Autodesk Inventor part; units mm, degrees
ref_plane "Arbeitsebene2" through (0, 0, 0) normal (1, 0, 0) x (0, 0, -1)
ref_plane "YZ Plane" through (0, 0, 0) normal (1, 0, 0) x (0, 1, 0)
ref_plane "XY Plane" through (0, 0, 0) normal (0, 0, 1) x (1, 0, 0)
sketch "Skizze1" plane through (0, 0, 0) normal (1, 0, 0) x (0, 1, 0)
  line L0 (-11, 0) -> (-6, 0)
  arc A0 (6, 0) -> (-6, 0) centre (0, 0) ccw
  line L1 (6, 0) -> (11, 0)
  line L2 (11, 0) -> (11, 8)
  line L3 (-11, 8) -> (-11, 0)
  line L4 (-11, 8) -> (11, 8)
  point P0 (0, 0)
  dimension "d2" = 6
  dimension "d18" = 22
  dimension "d26" = 8
extrude "Extrusion1" add sketch "Skizze1" along normal mid plane 5
ref_plane "Arbeitsebene2" through (0, 0, 0) normal (1, 0, 0) x (0, 0, -1)
sketch "Skizze5" plane through (2.5, -6, 0) normal (0, 0, -1) x (-1, 0, 0)
  line L0 (2.5, 6) -> (-2.4006, 6) construction
  line L1 (0, -5) -> (0, 0)
  point P0 (2.5, -2)
  point P1 (2.5, 14)
  dimension "d27" = 16
  dimension "d28" = 2.5
hole "Bohrung2" at (0, -8, 0) at (0, 8, 0) direction (0, 0, 1) diameter 3 end through all
chamfer "Fase1" distance 1 angle 45 4 edges at (0, -11, 8) (0, 11, 8) (0, 11, 0) (0, -11, 0)
properties part number "Halterung_Motor" material "ABS-Kunststoff"
For this review, take the finished solid that the model builds, in its own axes (mm). Round coordinates to 2 decimals unless told otherwise and drop trailing zeros. Order: outer loops, then holes, each group sorted by start corner. A loop starts at its lowest first (then second) coordinate and runs counter-clockwise, first axis right, second up. Notation, with made-up numbers: (12.25, 9.25) -> (60.25, 9.25) arc R28 ccw to (60.25, 35.25) -> close; hole circle Ø3 at (84.25, 66). An arc over 180 degrees is marked (long way). Write item = value, one per line. Start each with the question number.
1) The part is to be moulded in two halves that separate along Y. For faces 1 (the face through (0, -10.5, 0.5)), 2 (the face through (0, 0, 6)), 3 (the face through (-0.07, -9.5, 4.06)), 4 (the face through (-2.5, 0, 7)), say which applies: +Y half, -Y half, draft (parallel to the pull), parting line (faces both ways), or undercut.
2) Insertion check: pin 1 (1.8 mm diameter, centred on x = 0, y = -8, fed in from -Z). The pin has a flat end and moves straight along its axis. Give the tip position at first contact, or say it passes through.
3) Take a section at C-C on y = -8. State the section outline as (x, z) points, plus the area to 3 significant figures.
4) Take a section at D-D on x = 2. State the section outline as (y, z) points.
5) Take a section at B-B on z = 5.5. State the section outline as (x, y) points, plus the area to 3 significant figures.
6) To check wall thickness, follow line 1 (Y direction, x = 0, z = 6.25); line 2 (X direction, y = 8, z = 3.25); line 3 (Y direction, x = 0, z = 5.25). State the ranges of each line that lie inside material, in increasing order. Write a range as from..to.
7) Take a section at A-A on x = 0. State the section outline as (y, z) points, plus the area to 3 significant figures.
Verdict:
q1.face_1 = -Y half
q1.face_2 = undercut
q1.face_3 = undercut
q1.face_4 = draft
q2.pin_1 = through
q3.outline = (-2.5, 0) -> (-1.5, 0) -> (-1.5, 8) -> (-2.5, 8) -> close; (1.5, 0) -> (2.5, 0) -> (2.5, 8) -> (1.5, 8) -> close
q3.area = 16.0 mm2
q4.outline = (-11, 1) -> (-10, 0) -> (-6, 0) arc R6 cw to (6, 0) -> (10, 0) -> (11, 1) -> (11, 7) -> (10, 8) -> (-10, 8) -> (-11, 7) -> close
q5.outline = (-2.5, -11) -> (2.5, -11) -> (2.5, -2.4) -> (-2.5, -2.4) -> close; (-2.5, 2.4) -> (2.5, 2.4) -> (2.5, 11) -> (-2.5, 11) -> close; hole circle Ø3 at (0, -8); hole circle Ø3 at (0, 8)
q5.area = 71.9 mm2
q6.line_1 = -11..-9.5, -6.5..6.5, 9.5..11
q6.line_2 = -2.5..-1.5, 1.5..2.5
q6.line_3 = -11..-9.5, -6.5..-2.9, 2.9..6.5, 9.5..11
q7.outline = (-11, 1) -> (-10, 0) -> (-9.5, 0) -> (-9.5, 8) -> (-10, 8) -> (-11, 7) -> close; (-6.5, 0) -> (-6, 0) arc R6 cw to (6, 0) -> (6.5, 0) -> (6.5, 8) -> (-6.5, 8) -> close; (9.5, 0) -> (10, 0) -> (11, 1) -> (11, 7) -> (10, 8) -> (9.5, 8) -> close
q7.area = 69.5 mm2
